Part model, mm, in its own coordinate system. A direction names the side the tool comes from. Round coordinates to 2 decimals unless told otherwise and drop trailing zeros. Loops run counter-clockwise (first coordinate to the right, second up) from the corner with the lowest first, then second, coordinate; pieces in that order, holes last. Notation, with made-up numbers: M 70.25,29 L 85.25,29 A25 cw 85.25,68 Z; hole C 36,1 d10. An arc over 180 degrees is marked long. Write each question's results on one line, items separated by ' | '.
from build123d import *

# Parameters (mm, degrees)
PAD_DEPTH       = 35
PAD001_DEPTH    = 14.125
SKETCH006_R     = 5
POCKET_DEPTH    = 12
POCKET001_DEPTH = 2.5
FILLET_R        = 5


with BuildPart() as part:
    # Sketch → Pad (new body, symmetric)
    with BuildSketch(Plane.XZ):
        Polygon((0, 1.875), (-1.875, 0), (-1.875, 16), (1.875, 16), (1.875, 0), align=None)
    extrude(amount=PAD_DEPTH, both=True)

    # Sketch001 (on Face3 of Pad) → Pad001 (join)
    with BuildSketch(Plane(origin=(0, 0, 16), x_dir=(-1, 0, 0), z_dir=(0, 0, 1))):
        with BuildLine():
            ThreePointArc((6.35, 6), (0, 12.35), (-6.35, 6))
            Line((-6.35, 6), (-6.35, -6))
            ThreePointArc((-6.35, -6), (0, -12.35), (6.35, -6))
            Line((6.35, 6), (6.35, -6))
        make_face()
    extrude(amount=-PAD001_DEPTH)

    # Sketch006 (on Face15 of Pad001) → Pocket (cut)
    with BuildSketch(Plane(origin=(0, 0, 16), x_dir=(-1, 0, 0), z_dir=(0, 0, 1))):
        with Locations((0, 6)):
            Circle(SKETCH006_R)
        with Locations((0, -6)):
            Circle(SKETCH006_R)
    extrude(amount=-POCKET_DEPTH, mode=Mode.SUBTRACT)

    # Sketch005 → Pocket001 (cut, symmetric)
    with BuildSketch(Plane.YZ):
        Polygon((-36, 25), (-36, 1), (-12, 25), align=None)
        Polygon((12, 25), (36, 25), (36, 1), align=None)
    extrude(amount=POCKET001_DEPTH, both=True, mode=Mode.SUBTRACT)

    # Fillet
    fillet_edges = [part.edges().sort_by_distance(p)[0] for p in [
        (5, -6, 4),
        (5, 6, 4),
    ]]
    fillet(fillet_edges, radius=FILLET_R)


solid = part.part
Item 1: Which spindle directions (+Z, -Z, +X, -X, +Y, -Y) get a long thin tool onto all of the face, cutting with end or side? Do faces 4 (the flat face through (-4, 0, 1.875)), 5 (the flat face through (4, 0, 1.875)), 6 (the flat face through (0.951, -0.49, 0.924)). Say none if no direction does.
Filled sheet:
face 4: -Z, -X, +Y, -Y | face 5: -Z, +X, +Y, -Y | face 6: -Z, +Y, -Y
Item 2: Band-saw the part on A-A on z = 13.5. Give the cut face in (x, y) (3 decimals), and give its area (3 significant figures).
Filled sheet:
outline: M -6.35,-6 A6.35 ccw -1.875,-12.067 L -1.875,-23.5 L 1.875,-23.5 L 1.875,-12.067 A6.35 ccw 6.35,-6 L 6.35,6 A6.35 ccw 1.875,12.067 L 1.875,23.5 L -1.875,23.5 L -1.875,12.067 A6.35 ccw -6.35,6 Z; hole C 0,-6 d10; hole C 0,6 d10 | area: 206 mm^2
Item 3: Two-plate mould, pull along Y, no slides. Class faces 1 (the flat face through (0, 28, 9)), 2 (the flat face through (0, 0, 16)), 3 (the cylindrical face through (1.08, -1.12, 12.55)): +Y half, -Y half, draft (parallel to the pull), parting line (faces both ways), or undercut.
Filled sheet:
face 1: +Y half | face 2: draft | face 3: undercut
Item 4: Wall check: L1, parallel to X at y = -6, z = 10.75; L2, parallel to Y at x = 0, z = 13.5. Give the ranges that are in metal, low to high.
Filled sheet:
L1: -6.35 to -5, 5 to 6.35 | L2: -23.5 to -11, -1 to 1, 11 to 23.5
Item 5: Band-saw the part on B-B on y = -24. Give the cut face in (x, z) (3 decimals), and give its area (3 significant figures).
Filled sheet:
outline: M -1.875,0 L 0,1.875 L 1.875,0 L 1.875,13 L -1.875,13 Z | area: 45.2 mm^2
Item 6: Band-saw the part on D-D on z = 3. Give the cut face in (x, y) (3 decimals).
Filled sheet:
outline: M -6.35,-6 A6.35 ccw -1.875,-12.067 L -1.875,-34 L 1.875,-34 L 1.875,-12.067 A6.35 ccw 6.35,-6 L 6.35,6 A6.35 ccw 1.875,12.067 L 1.875,34 L -1.875,34 L -1.875,12.067 A6.35 ccw -6.35,6 Z
Item 7: Drop flat-ended pins along their axis: P1, Ø6, axis at y = 16, z = 12, coming from the +X side (3 decimals); P2, Ø2, axis at x = 4, y = -2.5, coming from the -Z side (3 decimals); P3, Ø1.5, axis at x = -2.5, z = 7.5, coming from the +Y side. Give the stop position or say it passes through.
Filled sheet:
P1: x = 1.875 | P2: z = 1.875 | P3: y = 29.91
Item 8: Band-saw the part on C-C on x = 1. Give the cut face in (y, z) (3 decimals).
Filled sheet:
outline: M -35,0.875 L 35,0.875 L 35,2 L 21,16 L 10.899,16 L 10.899,9 A4.899 cw 1.101,9 L 1.101,16 L -1.101,16 L -1.101,9 A4.899 cw -10.899,9 L -10.899,16 L -21,16 L -35,2 Z
